Can you work these out from the model? Positions are in its coordinate system, mm. A direction names the side the tool comes from. Coordinates: 2 decimals unless noted, no trailing zeros. Loops run counter-clockwise (first coordinate to the right, second up) from the corner with the lowest first, then second, coordinate; pieces in that order, holes last. Notation, with made-up numbers: (-4.5, -10.75) -> (29.5, -10.75) arc R28 ccw to (29.5, 8.25) -> close; hole circle Ø10 at (45, 26). An arc over 180 degrees is marked (long way). Put each result on its own line as item: value. Start each with the question number.
Item 1: Please list where these lines run through material, in increasing order: L1, parallel to X at y = 0.75, z = -0.5; L2, parallel to Z at x = -0.5, y = -0.9; L3, parallel to Z at x = -0.95, y = 0.5. Write a range as from..to.
Item 2: For faces 1 (the cylindrical face through (0, 1, 8)), 2 (the flat face through (0, -1, 0.25)), 3 (the cylindrical face through (0, 1, -8)), which set-ups out of +Z, -Z, +X, -X, +Y, -Y let a thin tool reach every point of the face, with its end or its side?
Item 3: If we section it at C-C on z = -3.25: Please give me the cut outline in (x, y).
Item 4: Will this pin go through, and if not, where does the flat tip stop? P1, Ø1.5, axis at x = 1.5, z = 3.5, coming from the +Y side.
Item 5: If we section it at B-B on x = 0: Please give me the cut outline in (y, z).
Item 6: If we section it at D-D on y = 1.3: Please give me the cut outline in (x, z).
Item 7: If we section it at A-A on y = 0: Please give me the cut outline in (x, z).
Autodesk Inventor part; units mm, degrees
ref_plane "Work Plane1" through (0, -1.75, 0) normal (0, 1, 0) x (-1, 0, 0)
ref_plane "YZ Plane" through (0, 0, 0) normal (1, 0, 0) x (0, 1, 0)
ref_plane "XY Plane" through (0, 0, 0) normal (0, 0, 1) x (1, 0, 0)
sketch "Sketch1" plane through (0, 0, 0) normal (0, 1, 0) x (-1, 0, 0)
  line L0 (0, 18.1135) -> (0, -15.5197) construction
  line L1 (0, 0) -> (5.9379, 0) construction
  line L2 (0, -8.5) -> (1, -8.5)
  line L3 (1, -8.5) -> (1, -7)
  line L4 (1, -7) -> (1.1561, -7)
  line L5 (1.5, -4.75) -> (1.75, -4.75)
  line L6 (1.75, -4.75) -> (1.75, 4.75)
  line L7 (1.75, 4.75) -> (1.5, 4.75)
  line L8 (1.5, 4.75) -> (1.5, 7)
  line L9 (1.5, 7) -> (1, 7)
  line L10 (1, 7) -> (1, 8.5)
  line L11 (1, 8.5) -> (0, 8.5)
  line L12 (0, -8.5) -> (0, 8.5)
  line L13 (1.5, -4.75) -> (1.5, -7)
  line L14 (1.5, -7) -> (1.1561, -7)
  dimension "d7" = 17
  dimension "d9" = 1
  dimension "d10" = 1.5
  dimension "d11" = 14
  dimension "d12" = 1.75
  dimension "d13" = 9.5
revolve "Revolution1" add sketch "Sketch1" angle 360 about axis through (0, 0, 18.1135) along (0, 0, -1)
ref_plane "Work Plane1" through (0, -1.75, 0) normal (0, 1, 0) x (-1, 0, 0)
sketch "Sketch2" plane through (0, -1.75, 0) normal (0, 1, 0) x (-1, 0, 0)
  line L0 (-1.75, -4.75) -> (1.75, -4.75)
  line L1 (-1.75, 4.75) -> (1.75, 4.75)
  line L2 (-1.75, -4.75) -> (1.75, -4.75)
  line L3 (-1.75, 4.75) -> (-1.75, -4.75)
  line L4 (1.75, 4.75) -> (1.75, -4.75)
  line L5 (-1.75, 0.25) -> (1.75, 0.25)
  line L6 (1.75, 0.25) -> (1.75, 8.5)
  line L7 (-1.75, 8.5) -> (-1.75, 0.25)
  line L8 (-1.5, 7) -> (1.5, 7)
  line L9 (-1.5, 4.75) -> (1.5, 4.75)
  line L10 (-1, 8.5) -> (1, 8.5)
  line L11 (-1.75, 8.5) -> (1.75, 8.5)
  dimension "d17" = 4.5
extrude "Extrusion1" cut sketch "Sketch2" along normal blind 1 contours L3 L1 L4 L5 | L7 L11 L10 L6 L1
properties part number "2nd_phalanx_shaft"
Solutions:
1. L1: -1.58..1.58
1. L2: -7..0.25
1. L3: -7..7
2. face 1: +Z
2. face 2: +Z, +X, -X, -Y
2. face 3: -Z
3. outline: circle Ø3.5 at (0, 0)
4. P1: y = 1.58
5. outline: (-1.75, -4.75) -> (-1.5, -4.75) -> (-1.5, -7) -> (-1, -7) -> (-1, -8.5) -> (1, -8.5) -> (1, -7) -> (1.5, -7) -> (1.5, -4.75) -> (1.75, -4.75) -> (1.75, 4.75) -> (1.5, 4.75) -> (1.5, 7) -> (1, 7) -> (1, 8.5) -> (-0.75, 8.5) -> (-0.75, 0.25) -> (-1.75, 0.25) -> close
6. outline: (-1.17, -4.75) -> (-0.75, -4.75) -> (-0.75, -7) -> (0.75, -7) -> (0.75, -4.75) -> (1.17, -4.75) -> (1.17, 4.75) -> (0.75, 4.75) -> (0.75, 7) -> (-0.75, 7) -> (-0.75, 4.75) -> (-1.17, 4.75) -> close
7. outline: (-1.75, -4.75) -> (-1.5, -4.75) -> (-1.5, -7) -> (-1, -7) -> (-1, -8.5) -> (1, -8.5) -> (1, -7) -> (1.5, -7) -> (1.5, -4.75) -> (1.75, -4.75) -> (1.75, 4.75) -> (1.5, 4.75) -> (1.5, 7) -> (1, 7) -> (1, 8.5) -> (-1, 8.5) -> (-1, 7) -> (-1.5, 7) -> (-1.5, 4.75) -> (-1.75, 4.75) -> close
